The model under review builds one solid part; all positions refer to its coordinate system, in mm. Face numbers are marked on the shaded views. A direction names the side the tool comes from. Coordinates: 2 decimals unless noted, no trailing zeros. Write each loop counter-clockwise with the first axis right and the second up, starting at its lowest first coordinate (ties: lowest second). Pieces come first, ordered by that corner, then holes. Notation, with made-up numbers: (55, 27) - (104, 27) arc R4 cw to (104, 33) - close; hole circle Ø6 at (-25.75, 65.25). An arc over 180 degrees is marked (long way). Put each result on its own line as item: value.
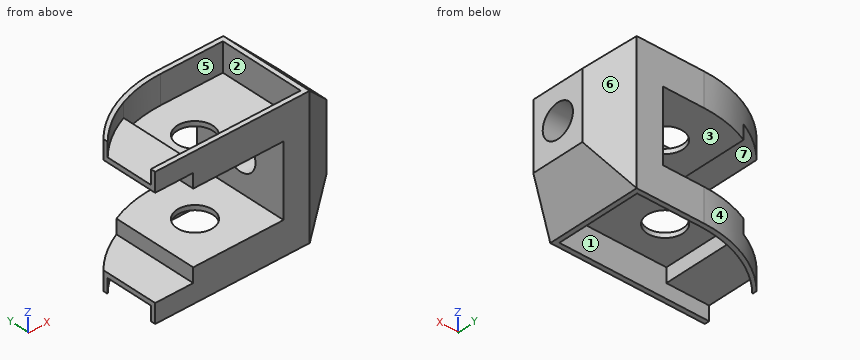
from build123d import *

# Parameters (mm, degrees)
SKETCH1_W           = 80
SKETCH1_H           = 58
BOSS_EXTRUDE1_DEPTH = 40
SKETCH2_R           = 7.5
CUT_EXTRUDE1_DEPTH  = 95
CUT_EXTRUDE4_DEPTH  = 95
SKETCH7_W           = 36.66060556
SKETCH7_H           = 15
SKETCH7_W_2         = 17.33939444
CUT_EXTRUDE5_DEPTH  = 95
SKETCH8_W           = 16
SKETCH8_H           = 42
CUT_EXTRUDE6_DEPTH  = 95
SKETCH9_R           = 7
CUT_EXTRUDE7_DEPTH  = 95
SKETCH15_R          = 7.5
CUT_EXTRUDE18_DEPTH = 12
CUT_EXTRUDE19_DEPTH = 6
CUT_EXTRUDE20_START = -12
SKETCH19_R          = 7.5
CUT_EXTRUDE20_DEPTH = 12
CUT_EXTRUDE21_START = -6
CUT_EXTRUDE21_DEPTH = 6


with BuildPart() as part:
    # Sketch1 → Boss-Extrude1 (new body)
    with BuildSketch(Plane(origin=(0, 0, 0), x_dir=(1, 0, 0), z_dir=(0, 1, 0))):
        Rectangle(SKETCH1_W, SKETCH1_H)
    extrude(amount=BOSS_EXTRUDE1_DEPTH)

    # Sketch2 → Cut-Extrude1 (cut)
    with BuildSketch(Plane.XY.offset(29)):
        with Locations((-6, 19)):
            Circle(SKETCH2_R)
        Polygon((25, 0), (40, 0), (40, 8.660254038), align=None)
        Polygon((25, 40), (40, 40), (40, 31.339745962), align=None)
    extrude(amount=-CUT_EXTRUDE1_DEPTH, mode=Mode.SUBTRACT)

    # Sketch4 → Cut-Extrude4 (cut)
    with BuildSketch(Plane.XY.offset(29)):
        with BuildLine():
            ThreePointArc((-40, 24), (-23.33939444, 35.82575695), (-3.33939444, 40))
            Line((-3.33939444, 40), (-40, 40))
            Line((-40, 40), (-40, 24))
        make_face()
    extrude(amount=-CUT_EXTRUDE4_DEPTH, mode=Mode.SUBTRACT)

    # Sketch7 → Cut-Extrude5 (cut)
    with BuildSketch(Plane(origin=(0, 40, 0), x_dir=(1, 0, 0), z_dir=(0, 1, 0))):
        with Locations((-21.66969722, -7.5)):
            Rectangle(SKETCH7_W, SKETCH7_H)
        with Locations((-21.66969722, 7.5)):
            Rectangle(SKETCH7_W, SKETCH7_H)
        with Locations((5.33030278, 7.5)):
            Rectangle(SKETCH7_W_2, SKETCH7_H)
        with Locations((5.33030278, -7.5)):
            Rectangle(SKETCH7_W_2, SKETCH7_H)
        Polygon((40, 14), (40, 29), (25, 29), align=None)
        Polygon((40, -29), (25, -29), (40, -14), align=None)
    extrude(amount=-CUT_EXTRUDE5_DEPTH, mode=Mode.SUBTRACT)

    # Sketch8 → Cut-Extrude6 (cut)
    with BuildSketch(Plane(origin=(0, 40, 0), x_dir=(1, 0, 0), z_dir=(0, 1, 0))):
        with Locations((-32, 0)):
            Rectangle(SKETCH8_W, SKETCH8_H)
    extrude(amount=-CUT_EXTRUDE6_DEPTH, mode=Mode.SUBTRACT)

    # Sketch9 → Cut-Extrude7 (cut)
    with BuildSketch(Plane(origin=(40, 0, 0), x_dir=(0, 0, -1), z_dir=(1, 0, 0))):
        with Locations((0, 20)):
            Circle(SKETCH9_R)
    extrude(amount=-CUT_EXTRUDE7_DEPTH, mode=Mode.SUBTRACT)

    # Sketch15 → Cut-Extrude18 (cut)
    with BuildSketch(Plane.XY.offset(29)):
        with BuildLine():
            Line((23, 2), (23, 38))
            Line((23, 38), (-3.339394, 38))
            ThreePointArc((-3.339394, 38), (-12.842943372, 37.088517575), (-22, 34.387302143))
            Line((-22, 34.387302143), (-22, 2))
            Line((-22, 2), (23, 2))
        make_face()
        with Locations((-6, 19)):
            Circle(SKETCH15_R, mode=Mode.SUBTRACT)
    extrude(amount=-CUT_EXTRUDE18_DEPTH, mode=Mode.SUBTRACT)

    # Sketch18 → Cut-Extrude19 (cut)
    with BuildSketch(Plane.XY.offset(29)):
        with BuildLine():
            Line((-22, 34.387302143), (-22, 2))
            Line((-22, 2), (-40, 2))
            Line((-40, 2), (-40, 22))
            ThreePointArc((-40, 22), (-31.684948122, 29.18894981), (-22, 34.387302143))
        make_face()
    extrude(amount=-CUT_EXTRUDE19_DEPTH, mode=Mode.SUBTRACT)

    # Sketch19 → Cut-Extrude20 (cut)
    with BuildSketch(Plane(origin=(0, 0, -29), x_dir=(-1, 0, 0), z_dir=(0, 0, -1)).offset(CUT_EXTRUDE20_START)):
        with BuildLine():
            Line((3.339394, 38), (-23, 38))
            Line((-23, 38), (-23, 2))
            Line((-23, 2), (22, 2))
            Line((22, 2), (22, 34.387302143))
            ThreePointArc((22, 34.387302143), (12.842943372, 37.088517575), (3.339394, 38))
        make_face()
        with Locations(Location((6, 19, 0), (0, 0, 180))):
            Circle(SKETCH19_R, mode=Mode.SUBTRACT)
    extrude(amount=CUT_EXTRUDE20_DEPTH, mode=Mode.SUBTRACT)

    # Sketch20 → Cut-Extrude21 (cut)
    with BuildSketch(Plane(origin=(0, 0, -29), x_dir=(-1, 0, 0), z_dir=(0, 0, -1)).offset(CUT_EXTRUDE21_START)):
        with BuildLine():
            Line((22, 34.387302143), (22, 2))
            Line((22, 2), (40, 2))
            Line((40, 2), (40, 22))
            ThreePointArc((40, 22), (31.684948122, 29.18894981), (22, 34.387302143))
        make_face()
    extrude(amount=CUT_EXTRUDE21_DEPTH, mode=Mode.SUBTRACT)


solid = part.part
1. The part is to be moulded in two halves that separate along X. For the marked faces 5, 6 and 7, say which applies: +X half, -X half, draft (parallel to the pull), parting line (faces both ways), or undercut.
Determined:
face 5: undercut
face 6: +X half
face 7: draft
2. To check wall thickness, follow probe 1 along Y at (x, z) = (20, 0); probe 2 along Z at (x, y) = (-5.5, 34); probe 3 along Z at (x, y) = (-30.5, 17). State the ranges of each line that lie inside material, in increasing order.
Determined:
probe 1: y = 0 to 13, 27 to 40
probe 2: z = -17 to -15, 15 to 17
probe 3: z = -23 to -21, 21 to 23
3. Consider section D-D on x = -6. State the section outline as (y, z) points.
Determined:
outline: (0, -29) - (2, -29) - (2, -17) - (11.5, -17) - (11.5, -15) - (0, -15) - close; (0, 15) - (11.5, 15) - (11.5, 17) - (2, 17) - (2, 29) - (0, 29) - close; (26.5, -17) - (37.93, -17) - (37.93, -29) - (39.93, -29) - (39.93, -15) - (26.5, -15) - close; (26.5, 15) - (39.93, 15) - (39.93, 29) - (37.93, 29) - (37.93, 17) - (26.5, 17) - close
4. Consider section C-C on y = 19. Give the number of separate pieces and of enclosed holes in the cut face, plus the area to 3 significant figures.
Determined:
separate pieces: 4
enclosed holes: 0
area: 887 mm^2
5. Consider section A-A on x = 10.5. State the section outline as (y, z) points.
Determined:
outline: (0, -29) - (2, -29) - (2, -17) - (38, -17) - (38, -29) - (40, -29) - (40, -15) - (0, -15) - close; (0, 15) - (40, 15) - (40, 29) - (38, 29) - (38, 17) - (2, 17) - (2, 29) - (0, 29) - close
6. For pin 1 Ø11 at (x, y) = (2, 14) entering from -Z; pin 2 Ø18 at (x, y) = (0.5, 24) entering from +Z; pin 3 Ø1.5 at (y, z) = (17, 21) entering from +X; pin 4 Ø1 at (x, z) = (-22.5, -14) entering from +Y, all flat-tipped, find the tip position at first contact; note any pin that passes through.
Determined:
pin 1: stops at z = -17
pin 2: stops at z = 17
pin 3: stops at x = 33.75
pin 4: passes through
7. Consider section B-B on z = 0. State the section outline as (x, y) points.
Determined:
outline: (14, 0) - (25, 0) - (40, 8.66) - (40, 13) - (14, 13) - close; (14, 27) - (40, 27) - (40, 31.34) - (25, 40) - (14, 40) - close
8. Machinability: for the marked faces 1, 2, 3 and 4, which of the approach directions +Z, -Z, +X, -X, +Y, -Y give a long, thin tool a straight path to every point of the face, cutting with its end or side? Answer none if there is none.
Determined:
face 1: -Z
face 2: +Z
face 3: -X, +Y, -Y
face 4: +Z, -Z, -X, +Y
